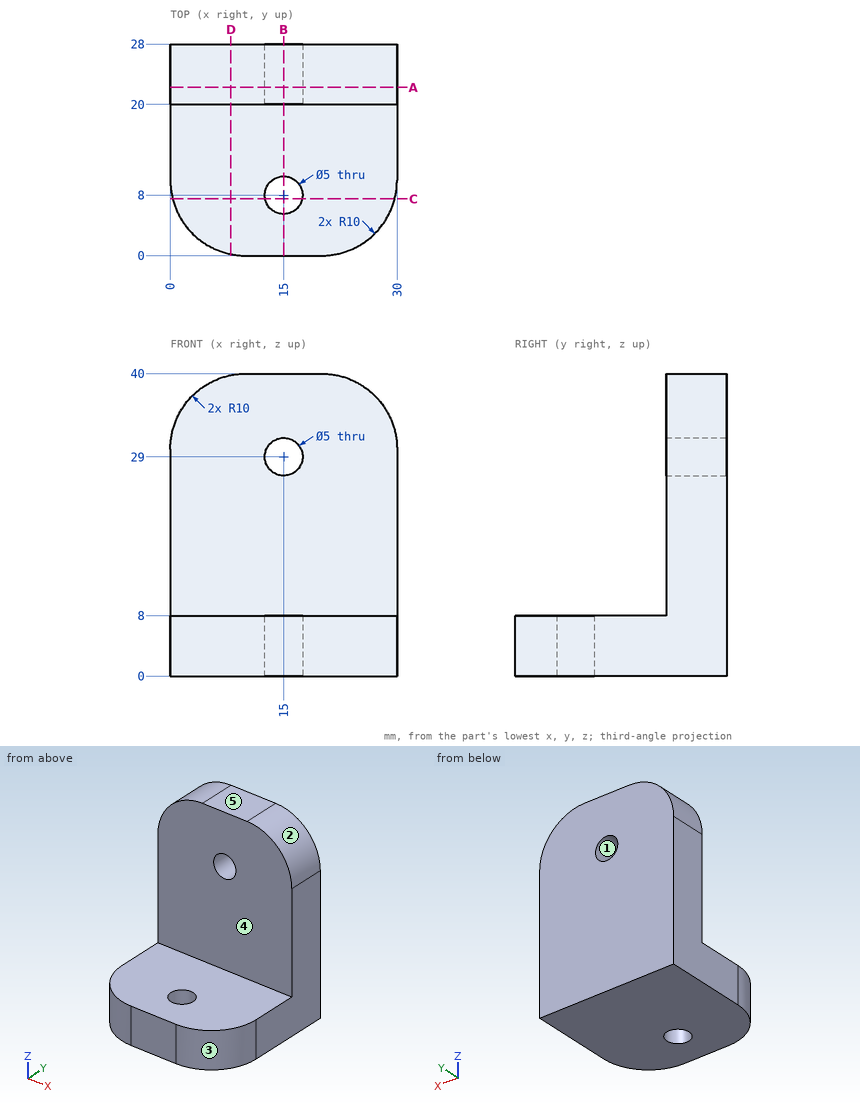
The drawing under review shows one solid part. Ordinate dimensions are in mm from its lowest x, y, z. A direction names the side the tool comes from. Coordinates: 2 decimals unless noted, no trailing zeros. Write each loop counter-clockwise with the first axis right and the second up, starting at its lowest first coordinate (ties: lowest second). Pieces come first, ordered by that corner, then holes.
1) Add section D-D (x = 8). Write out the cut boundary in (y, z), plus the area to 3 significant figures.
2) To check wall thickness, follow L1, parallel to Y at x = 15, z = 4.5; L2, parallel to Z at x = 15, y = 24; L3, parallel to X at y = 24.5, z = 29. State the ranges of each line that lie inside material, in increasing order.
3) Mouldability with a two-part tool opening along Z and no side actions: class the marked faces 1, 2 and 3 as +Z half, -Z half, draft (parallel to the pull), parting line (faces both ways), or undercut.
4) Insertion check: pin 1 (10 mm diameter, centred on x = 25.5, z = 9, fed in from -Y); pin 2 (5 mm diameter, centred on x = 6, z = 33.5, fed in from -Y); pin 3 (12 mm diameter, centred on y = 18, z = 31.5, fed in from -X); pin 4 (8 mm diameter, centred on x = 4.5, y = 7, fed in from +Z). Each pin has a flat end and moves straight along its axis. Give the tip position at first contact, or say it passes through.
5) Add section C-C (y = 7.5). Write out the cut boundary in (x, z).
6) Machinability: for the marked faces 4 and 5, which of the approach directions +Z, -Z, +X, -X, +Y, -Y give a long, thin tool a straight path to every point of the face, cutting with its end or side? Answer none if there is none.
7) Add section B-B (x = 15). Write out the cut boundary in (y, z), plus the area to 3 significant figures.
8) Add section A-A (y = 22.25). Write out the cut boundary in (x, z).
Check result:
1. outline: (0.2, 0) - (28, 0) - (28, 39.8) - (20, 39.8) - (20, 8) - (0.2, 8) - close
1. area: 477 mm2
2. L1: y = 0 to 5.5, 10.5 to 28
2. L2: z = 0 to 26.5, 31.5 to 40
2. L3: x = 0 to 12.5, 17.5 to 30
3. face 1: undercut
3. face 2: +Z half
3. face 3: draft
4. pin 1: stops at y = 0.02
4. pin 2: stops at y = 20
4. pin 3: stops at x = 0
4. pin 4: stops at z = 8
5. outline: (0.32, 0) - (12.55, 0) - (12.55, 8) - (0.32, 8) - close; (17.45, 0) - (29.68, 0) - (29.68, 8) - (17.45, 8) - close
6. face 4: +Z, +X, -X, -Y
6. face 5: +Z, +X, -X, +Y, -Y
7. outline: (0, 0) - (5.5, 0) - (5.5, 8) - (0, 8) - close; (10.5, 0) - (28, 0) - (28, 26.5) - (20, 26.5) - (20, 8) - (10.5, 8) - close; (20, 31.5) - (28, 31.5) - (28, 40) - (20, 40) - close
7. area: 400 mm2
8. outline: (0, 0) - (30, 0) - (30, 30) arc R10 ccw to (20, 40) - (10, 40) arc R10 ccw to (0, 30) - close; hole circle Ø5 at (15, 29)
